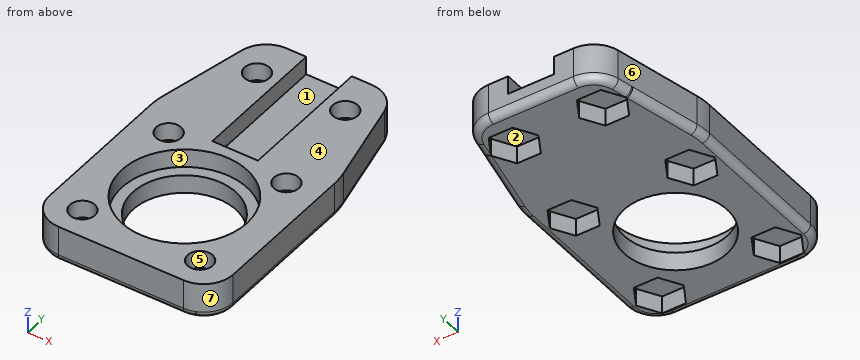
from build123d import *

# Parameters (mm, degrees)
SKETCH_R        = 7
PAD_DEPTH       = 5
SKETCH001_R     = 8.5
SKETCH001_W     = 6.2
SKETCH001_H     = 20
POCKET_DEPTH    = 2.5
FILLET_R        = 4
FILLET001_R     = 4
POCKET001_DEPTH = 2.4
SKETCH003_R     = 1.7
POCKET002_DEPTH = 2.4
FILLET002_R     = 4
FILLET003_R     = 4
FILLET004_R     = 10
FILLET005_R     = 10
FILLET006_R     = 1


with BuildPart() as part:
    # Sketch → Pad (new body)
    with BuildSketch(Plane.XY):
        Polygon((-12.5, -12.5), (12.5, -12.5), (12.5, 12.5), (9, 28.5), (-9, 28.5), (-12.5, 12.5), align=None)
        Circle(SKETCH_R, mode=Mode.SUBTRACT)
    extrude(amount=PAD_DEPTH)

    # Sketch001 → Pocket (cut)
    with BuildSketch(Plane.XY.offset(5)):
        Circle(SKETCH001_R)
        with Locations((0, 20)):
            Rectangle(SKETCH001_W, SKETCH001_H)
    extrude(amount=-POCKET_DEPTH, mode=Mode.SUBTRACT)

    # Fillet
    fillet_edges = [part.edges().sort_by_distance(p)[0] for p in [
        (-12.5, -12.5, 2.5),
    ]]
    fillet(fillet_edges, radius=FILLET_R)

    # Fillet001
    fillet001_edges = [part.edges().sort_by_distance(p)[0] for p in [
        (12.5, -12.5, 2.5),
    ]]
    fillet(fillet001_edges, radius=FILLET001_R)

    # Sketch002 → Pocket001 (cut)
    with BuildSketch(Plane(origin=(0, 0, 0), x_dir=(1, 0, 0), z_dir=(0, 0, -1))):
        Polygon((-9.616581, 11.3), (-11.233162, 8.5), (-9.616581, 5.7), (-6.383419, 5.7), (-4.766838, 8.5), (-6.383419, 11.3), align=None)
        Polygon((6.383419, 11.3), (4.766838, 8.5), (6.383419, 5.7), (9.616581, 5.7), (11.233162, 8.5), (9.616581, 11.3), align=None)
        Polygon((-9.616581, -5.7), (-11.233162, -8.5), (-9.616581, -11.3), (-6.383419, -11.3), (-4.766838, -8.5), (-6.383419, -5.7), align=None)
        Polygon((6.383419, -5.7), (4.766838, -8.5), (6.383419, -11.3), (9.616581, -11.3), (11.233162, -8.5), (9.616581, -5.7), align=None)
        Polygon((-7.616581, -20.2), (-9.233162, -23), (-7.616581, -25.8), (-4.383419, -25.8), (-2.766838, -23), (-4.383419, -20.2), align=None)
        Polygon((4.383419, -20.2), (2.766838, -23), (4.383419, -25.8), (7.616581, -25.8), (9.233162, -23), (7.616581, -20.2), align=None)
    extrude(amount=-POCKET001_DEPTH, mode=Mode.SUBTRACT)

    # Sketch003 → Pocket002 (cut)
    with BuildSketch(Plane.XY.offset(5)):
        with Locations((-8, 8.5)):
            Circle(SKETCH003_R)
        with Locations((8, 8.5)):
            Circle(SKETCH003_R)
        with Locations((-8, -8.5)):
            Circle(SKETCH003_R)
        with Locations((8, -8.5)):
            Circle(SKETCH003_R)
        with Locations((-6, 23)):
            Circle(SKETCH003_R)
        with Locations((6, 23)):
            Circle(SKETCH003_R)
    extrude(amount=-POCKET002_DEPTH, mode=Mode.SUBTRACT)

    # Fillet002
    fillet002_edges = [part.edges().sort_by_distance(p)[0] for p in [
        (9, 28.5, 2.5),
    ]]
    fillet(fillet002_edges, radius=FILLET002_R)

    # Fillet003
    fillet003_edges = [part.edges().sort_by_distance(p)[0] for p in [
        (-9, 28.5, 2.5),
    ]]
    fillet(fillet003_edges, radius=FILLET003_R)

    # Fillet004
    fillet004_edges = [part.edges().sort_by_distance(p)[0] for p in [
        (12.5, 12.5, 2.5),
    ]]
    fillet(fillet004_edges, radius=FILLET004_R)

    # Fillet005
    fillet005_edges = [part.edges().sort_by_distance(p)[0] for p in [
        (-12.5, 12.5, 2.5),
    ]]
    fillet(fillet005_edges, radius=FILLET005_R)

    # Fillet006
    fillet006_edges = [part.edges().sort_by_distance(p)[0] for p in [
        (-12.5, 1.459515, 0),
    ]]
    fillet(fillet006_edges, radius=FILLET006_R)


solid = part.part
Can you work these out from the model? Positions are in its coordinate system, mm. Face numbers are marked on the shaded views. A direction names the side the tool comes from. Give positions to 0.01 mm unless a question says otherwise; leave off trailing zeros. Loops run counter-clockwise (first coordinate to the right, second up) from the corner with the lowest first, then second, coordinate; pieces in that order, holes last. Notation, with made-up numbers: (61.25, 49) -> (91.25, 49) arc R20 ccw to (91.25, 59) -> close; hole circle Ø5 at (20, 62). An arc over 180 degrees is marked (long way). Write item = value, one per line.
1) Suppose I cut it at D-D on z = 1.65. Give the number of separate pieces and of enclosed holes in the cut face, then the cut area to 3 significant figures.
Check result:
separate_pieces = 1
enclosed_holes = 7
area = 641 mm2
2) Suppose I cut it at C-C on x = 0. Write out the boundary of the cut face in (y, z).
Check result:
outline = (-12.5, 1) arc R1 ccw to (-11.5, 0) -> (-7, 0) -> (-7, 2.5) -> (-8.5, 2.5) -> (-8.5, 5) -> (-12.5, 5) -> close; (7, 0) -> (27.5, 0) arc R1 ccw to (28.5, 1) -> (28.5, 2.5) -> (10, 2.5) -> (10, 5) -> (8.5, 5) -> (8.5, 2.5) -> (7, 2.5) -> close
3) Suppose I cut it at B-B on z = 3.65. Write out the boundary of the cut face in (x, y), then the cut area to 3 significant figures.
Check result:
outline = (-12.5, -8.5) arc R4 ccw to (-8.5, -12.5) -> (8.5, -12.5) arc R4 ccw to (12.5, -8.5) -> (12.5, 11.42) arc R10 ccw to (12.27, 13.56) -> (9.69, 25.35) arc R4 ccw to (5.78, 28.5) -> (3.1, 28.5) -> (3.1, 10) -> (-3.1, 10) -> (-3.1, 28.5) -> (-5.78, 28.5) arc R4 ccw to (-9.69, 25.35) -> (-12.27, 13.56) arc R10 ccw to (-12.5, 11.42) -> close; hole circle Ø3.4 at (-8, -8.5); hole circle Ø3.4 at (-8, 8.5); hole circle Ø17 at (0, 0); hole circle Ø3.4 at (-6, 23); hole circle Ø3.4 at (6, 23); hole circle Ø3.4 at (8, -8.5); hole circle Ø3.4 at (8, 8.5)
area = 562 mm2
4) Suppose I cut it at A-A on y = 0. Write out the boundary of the cut face in (x, z).
Check result:
outline = (-12.5, 1) arc R1 ccw to (-11.5, 0) -> (-7, 0) -> (-7, 2.5) -> (-8.5, 2.5) -> (-8.5, 5) -> (-12.5, 5) -> close; (7, 0) -> (11.5, 0) arc R1 ccw to (12.5, 1) -> (12.5, 5) -> (8.5, 5) -> (8.5, 2.5) -> (7, 2.5) -> close
5) For the marked faces 1, 2 and 3, which set-ups out of +Z, -Z, +X, -X, +Y, -Y let a thin tool reach every point of the face, with its end or its side?
Check result:
face_1 = +Z, +Y
face_2 = -Z
face_3 = +Z
6) Thinking about a two-plate mould opening in Y: for the marked faces 4, 5, 6 and 7, which applies, released by +Y, released by -Y, zero draft, split by the parting line, or undercut?
Check result:
face_4 = zero draft
face_5 = undercut
face_6 = released by +Y
face_7 = released by -Y
7) I need wall thicknesses on L1, parallel to Y at x = 0, z = 1.8; L2, parallel to X at y = 21.5, z = 3.65; L3, parallel to Y at x = 6, z = 3.8. Which ranges of each line are inside material? Lowest first, please. Write a range as from..to.
Check result:
L1 = -12.5..-7, 7..28.5
L2 = -10.53..-6.8, -5.2..-3.1, 3.1..5.2, 6.8..10.53
L3 = -12.5..-6.02, 6.02..21.3, 24.7..28.49
8) Will these pins go through, and if not, where does the flat tip stop? pin 1 (1.9 mm diameter, centred on x = -7.5, z = 2, fed in from +Y); pin 2 (2 mm diameter, centred on y = 23.5, z = 4, fed in from +X); pin 3 (1.2 mm diameter, centred on x = 7.5, z = 1, fed in from +Y).
Check result:
pin_1 = 28.43
pin_2 = 10.31
pin_3 = 28.34
